```python
from build123d import *

# Parameters (mm, degrees)
SKETCH_1_W                = 20
SKETCH_1_H                = 20
EXTRUDE_1_DEPTH           = 50.534412113
SKETCH_7_W                = 21.267206056
SKETCH_7_H                = 10
CUT_EXTRUDE_6_DEPTH       = 34
SKETCH_3_R                = 4.5
CUT_EXTRUDE_2_DEPTH       = 21
SKETCH_2_R                = 6.5
CUT_EXTRUDE_9_DEPTH       = 5
MOVE_BODY_1_ANGLE         = 90
SKETCH_8_W                = 20
SKETCH_8_H                = 20
EXTRUDE_2_DEPTH           = 8
SKETCH_9_W                = 14
SKETCH_9_H                = 4
CUT_EXTRUDE_10_DEPTH      = 15
CUT_EXTRUDE_11_DEPTH      = 49
CUT_EXTRUDE_11_DEPTH_BACK = 49
SKETCH_10_R               = 1.25


# Read off the part's stored shape, not the designer's step: the other step
with BuildPart() as part:
    # Sketch 1 → Extrude 1 (new body)
    with BuildSketch(Plane.XY):
        Rectangle(SKETCH_1_W, SKETCH_1_H)
    extrude(amount=EXTRUDE_1_DEPTH)

    # Sketch 7 → Cut-Extrude 6 (cut)
    with BuildSketch(Plane(origin=(10, 0, 0), x_dir=(0, 0, -1), z_dir=(1, 0, 0))):
        with Locations((-10.633603028, 5)):
            Rectangle(SKETCH_7_W, SKETCH_7_H)
    cut_extrude_6 = extrude(amount=-CUT_EXTRUDE_6_DEPTH, mode=Mode.SUBTRACT)

    # Sketch 3 → Cut-Extrude 2 (cut)
    with BuildSketch(Plane(origin=(0, -10, 0), x_dir=(-1, 0, 0), z_dir=(0, -1, 0))):
        with Locations(Location((0, -11.267206056, 0), (0, 0, 90))):
            Circle(SKETCH_3_R)
        with BuildLine():
            Line((-21.262122506, -11.267206056), (-9.5, -11.267206056))
            ThreePointArc((-9.5, -11.267206056), (0, -1.767206056), (9.5, -11.267206056))
            Line((9.5, -11.267206056), (21.262122506, -11.267206056))
            ThreePointArc((21.262122506, -11.267206056), (0, 9.99491645), (-21.262122506, -11.267206056))
        make_face()
    cut_extrude_2 = extrude(amount=-CUT_EXTRUDE_2_DEPTH, mode=Mode.SUBTRACT)

    # Sketch 2 → Cut-Extrude 9 (cut)
    with BuildSketch(Plane(origin=(0, -10, 0), x_dir=(-1, 0, 0), z_dir=(0, -1, 0))):
        with Locations(Location((0, -11.267206056, 0), (0, 0, 90))):
            Circle(SKETCH_2_R)
    cut_extrude_9 = extrude(amount=-CUT_EXTRUDE_9_DEPTH, mode=Mode.SUBTRACT)

    # Mirror 6: Cut-Extrude 6, Cut-Extrude 2, Cut-Extrude 9 across plane
    add(cut_extrude_6.mirror(Plane.XY.offset(25.267206056)), mode=Mode.SUBTRACT)
    add(cut_extrude_2.mirror(Plane.XY.offset(25.267206056)), mode=Mode.SUBTRACT)
    add(cut_extrude_9.mirror(Plane.XY.offset(25.267206056)), mode=Mode.SUBTRACT)


with BuildPart() as body_2:
    # Other 3: the piece on the far side of the plane
    add(part.part)
    split(bisect_by=Plane.XY.offset(25.267206056), keep=Keep.BOTTOM)


with BuildPart() as part_1:
    add(part.part)

    # Other 3
    split(bisect_by=Plane.XY.offset(25.267206056), keep=Keep.TOP)


with BuildPart() as part_2:
    # Move Body 1: moved
    add(part_1.part.rotate(Axis((0, 0, 0), (0, 0, 1)), MOVE_BODY_1_ANGLE))


    add(body_2.part)  # Extrude 2 merges body 2
    # Sketch 8 → Extrude 2 (add)
    with BuildSketch(Plane.XY.offset(21.267206056)):
        Rectangle(SKETCH_8_W, SKETCH_8_H)
    extrude(amount=EXTRUDE_2_DEPTH)

    # Sketch 9 → Cut-Extrude 10 (cut)
    with BuildSketch(Plane.XZ.offset(10)):
        with Locations((0, 25.267206056)):
            Rectangle(SKETCH_9_W, SKETCH_9_H)
    extrude(amount=-CUT_EXTRUDE_10_DEPTH, mode=Mode.SUBTRACT)

    # Sketch 10 → Cut-Extrude 11 (cut, two sides: drawn at the far end of the back side and taken through both)
    with BuildSketch(Plane.ZY.offset(-7).offset(-CUT_EXTRUDE_11_DEPTH_BACK)):
        with Locations((25.267206056, -6)):
            Circle(SKETCH_10_R)
        with Locations((25.267206056, 1)):
            Circle(SKETCH_10_R)
    extrude(amount=CUT_EXTRUDE_11_DEPTH + CUT_EXTRUDE_11_DEPTH_BACK, mode=Mode.SUBTRACT)


solid = part_2.part
```
CAD build for the part. Positions are in the model's coordinates, mm. A direction names the side the tool comes from. Coordinates: 2 decimals unless noted, no trailing zeros. Order: outer loops, then holes, each group sorted by start corner. A loop starts at its lowest first (then second) coordinate and runs counter-clockwise, first axis right, second up. Notation, with made-up numbers: (1.5, 7.25) - (6.5, 7.25) arc R24 ccw to (6.5, 33.25) - close; hole circle Ø3 at (0.25, 57). An arc over 180 degrees is marked (long way). Answer in a Markdown table with one row per item.
1. Slice it at B-B, the plane x = 1.25. List the corners of the cut face in (y, z).
Answer:
| item | result |
|---|---|
| outline | (-10, 1.85) - (0, 1.85) - (0, 6.94) - (-5, 6.94) - (-5, 4.89) - (-10, 4.89) - close; (-10, 17.65) - (-5, 17.65) - (-5, 15.59) - (0, 15.59) - (0, 21.27) - (10, 21.27) - (10, 39.27) - (9.5, 39.27) arc R9.5 ccw to (-9.5, 39.27) - (-10, 39.27) - (-10, 27.27) - (5, 27.27) - (5, 23.27) - (-10, 23.27) - close; hole circle Ø9 at (0, 39.27) |
2. 3-axis set-ups, long thin cutter, end or side, ignore diameter. For faces 5 (the face through (7.535, 1.952, 45.467)), 6 (the face through (-5, 0, 29.267)), 7 (the face through (2, -5, 7)), 8 (the face through (8.52, 0.52, 26.42)), 9 (the face through (0, 5, 21.267)): which of +Z, -Z, +X, -X, +Y, -Y reach the whole face in a straight line?
Answer:
| item | result |
|---|---|
| face 5 | +X |
| face 6 | +Z, -X, +Y, -Y |
| face 7 | -Y |
| face 8 | +X, -X |
| face 9 | -Z, +X, -X, +Y |
3. Slice it at D-D, the plane z = 40. List the corners of the cut face in (x, y).
Answer:
| item | result |
|---|---|
| outline | (0, -9.47) - (10, -9.47) - (10, -6.46) - (5, -6.46) - (5, -4.44) - (0, -4.44) - close; (0, 4.44) - (5, 4.44) - (5, 6.46) - (10, 6.46) - (10, 9.47) - (0, 9.47) - close |
4. Flat gauge pins, fed straight in: P1, Ø3, axis at y = 1, z = 25.27, coming from the -X side; P2, Ø8, axis at x = -5.5, y = 5, coming from the +Z side; P3, Ø1.5, axis at x = -4.5, y = -3, coming from the -Z side; P4, Ø2, axis at y = -6, z = 25.27, coming from the -X side. Where does each tip first touch, or does it go through?
Answer:
| item | result |
|---|---|
| P1 | x = -10 |
| P2 | z = 29.27 |
| P3 | z = 2.54 |
| P4 | through |
5. Pull direction X, two halves, no side cores. Call faces 1 (the face through (0.21, -5.07, 1.77)), 2 (the face through (-8.48, 0.52, 26.42)), 3 (the face through (7, -3, 25)), 4 (the face through (0, -3, 27.267)): +X half, -X half, draft (parallel to the pull), parting line (faces both ways), or undercut.
Answer:
| item | result |
|---|---|
| face 1 | parting line |
| face 2 | draft |
| face 3 | undercut |
| face 4 | undercut |
6. Slice it at C-C, the plane y = -2.5. List the corners of the cut face in (x, z).
Answer:
| item | result |
|---|---|
| outline | (-10, 11.27) - (-9.5, 11.27) arc R9.5 ccw to (9.5, 11.27) - (10, 11.27) - (10, 33.27) - (5, 33.27) - (5, 35.53) - (0, 35.53) - (0, 29.27) - (-10, 29.27) - close; (0, 43.01) - (5, 43.01) - (5, 45.27) - (10, 45.27) - (10, 48.43) - (0, 48.43) - close; hole (-7, 23.27) - (7, 23.27) - (7, 27.27) - (-7, 27.27) - close; hole circle Ø9 at (0, 11.27) |
7. Slice it at A-A, the plane y = -6. List the corners of the cut face in (x, z).
Answer:
| item | result |
|---|---|
| outline | (-10, 11.27) - (-9.5, 11.27) arc R9.5 ccw to (9.5, 11.27) - (10, 11.27) - (10, 24.02) - (7, 24.02) - (7, 23.27) - (-7, 23.27) - (-7, 24.02) - (-10, 24.02) - close; (-10, 26.52) - (-7, 26.52) - (-7, 27.27) - (7, 27.27) - (7, 26.52) - (10, 26.52) - (10, 36.77) - (5, 36.77) - (5, 41.77) - (10, 41.77) - (10, 46.63) - (0, 46.63) - (0, 29.27) - (-10, 29.27) - close; hole circle Ø13 at (0, 11.27) |
8. Drill centre lines: L1, parallel to Y at x = 4.75, z = 39.5; L2, parallel to Z at x = -2.25, y = 3.5; L3, parallel to Z at x = -1.25, y = -7.5. Where is each one in solid material? Low to high. Write a range as from..to.
Answer:
| item | result |
|---|---|
| L1 | -9.5..-4.49, 4.49..9.5 |
| L2 | 21.27..23.27, 27.27..29.27 |
| L3 | 1.85..4.89, 17.65..23.27, 27.27..29.27 |
